from build123d import *

# Parameters (mm, degrees)
F1_DEPTH    = 10
F2_T1_DEPTH = 10
F2_T3_DEPTH = 20


# Not quite as in the source:
# - a fillet or chamfer that OpenCascade refuses, or shapes differently, is made with other operations: its cross-section is extruded or revolved along the edge and cut away or added
# - a feature names something its author has since deleted; it is built from what else it names


with BuildPart() as f1:
    # F0 (on Right) → F1 (new body)
    with BuildSketch(Plane.YZ):
        with BuildLine():
            Line((20, 0), (0, 0))
            Line((0, 0), (0, -3))
            Line((0, -3), (15, -3))
            ThreePointArc((15, -3), (36.9203102168, 6.0796897832), (46, 28))
            ThreePointArc((46, 28), (44.5, 29.5), (43, 28))
            ThreePointArc((43, 28), (37.1421356237, 13.8578643763), (23, 8))
            Line((23, 8), (23, 18))
            ThreePointArc((23, 18), (21.5, 19.5), (20, 18))
            Line((20, 18), (20, 8))
            Line((20, 8), (0, 8))
            Line((0, 8), (0, 5))
            Line((0, 5), (20, 5))
            Line((20, 5), (20, 0))
        make_face()
        with BuildLine():
            Line((23, 0.1252802705), (23, 6))
            ThreePointArc((23, 6), (30.9268806632, 7.4777057094), (37.7888888889, 11.712312459))
            ThreePointArc((37.7888888889, 11.712312459), (38.4580316617, 11.7150853421), (38.5307017544, 11.0498945447))
            ThreePointArc((38.5307017544, 11.0498945447), (31.6848160775, 4.2804529457), (23, 0.1252802705))
        make_face(mode=Mode.SUBTRACT)
    extrude(amount=F1_DEPTH)

    # F2: fillet of radius 2 on 8 edges, made by hand

    # F2_s2 → F2_t1 (join)
    with BuildSketch(Plane.YZ):
        with BuildLine():
            ThreePointArc((20, 10), (19.4142135624, 8.5857864376), (18, 8))
            Line((18, 8), (20, 8))
            Line((20, 8), (20, 10))
        make_face()
        with BuildLine():
            ThreePointArc((25.2222222222, 8.1238402), (23.6666666667, 8.620744195), (23, 10.11145618))
            Line((23, 10.11145618), (23, 8))
            ThreePointArc((23, 8), (24.1128351181, 8.0309840503), (25.2222222222, 8.1238402))
        make_face()
        with BuildLine():
            ThreePointArc((23, 4.0834785138), (23.5280398556, 5.4374849146), (24.8333333333, 6.076521971))
            ThreePointArc((24.8333333333, 6.076521971), (23.9174648117, 6.0191388176), (23, 6))
            Line((23, 6), (23, 4.0834785138))
        make_face()
        with BuildLine():
            ThreePointArc((25.7407407407, 1.0623592655), (23.8778327846, 1.2646093225), (23, 2.920127592))
            Line((23, 2.920127592), (23, 0.1252802705))
            ThreePointArc((23, 0.1252802705), (24.3820770695, 0.5595803629), (25.7407407407, 1.0623592655))
        make_face()
    extrude(amount=F2_T1_DEPTH)

    # F2_s4 → F2_t3 (cut)
    with BuildSketch(Plane.YZ.offset(-5)):
        with BuildLine():
            ThreePointArc((2, 8), (0.5857864376, 7.4142135624), (0, 6))
            Line((0, 6), (0, 8))
            Line((0, 8), (2, 8))
        make_face()
        with BuildLine():
            ThreePointArc((0, 7), (0.5857864376, 5.5857864376), (2, 5))
            Line((2, 5), (0, 5))
            Line((0, 5), (0, 7))
        make_face()
        with BuildLine():
            ThreePointArc((2, 0), (0.5857864376, -0.5857864376), (0, -2))
            Line((0, -2), (0, 0))
            Line((0, 0), (2, 0))
        make_face()
        with BuildLine():
            ThreePointArc((0, -1), (0.5857864376, -2.4142135624), (2, -3))
            Line((2, -3), (0, -3))
            Line((0, -3), (0, -1))
        make_face()
    extrude(amount=F2_T3_DEPTH, mode=Mode.SUBTRACT)


solid = f1.part
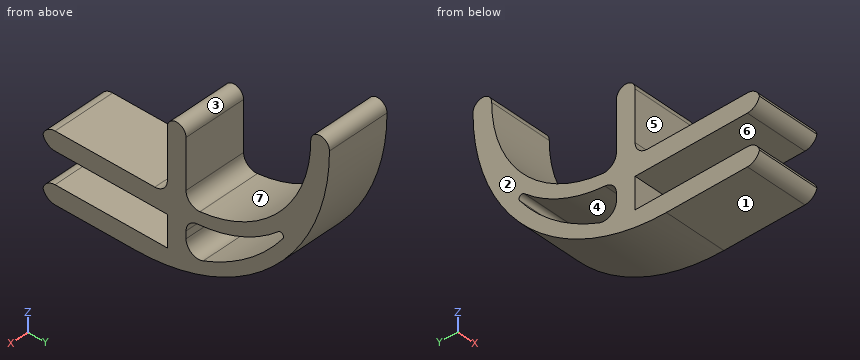
Part model, mm, in its own coordinate system. Face numbers are marked on the shaded views. A direction names the side the tool comes from. Give positions to 0.01 mm unless a question says otherwise; leave off trailing zeros. Order: outer loops, then holes, each group sorted by start corner. A loop starts at its lowest first (then second) coordinate and runs counter-clockwise, first axis right, second up. Notation, with made-up numbers: (36.5, 10.5) -> (75.5, 10.5) arc R21 ccw to (75.5, 21.5) -> close; hole circle Ø6 at (-4, -18). An arc over 180 degrees is marked (long way). Use one line per item in the form item = value.
(1) Saw through at C-C (z = 9.5). Write the cut outline in (x, y), then the cut area to 3 significant figures.
Solution:
outline = (0, 19.94) -> (10, 19.94) -> (10, 23.1) -> (0, 23.1) -> close; (0, 30.6) -> (10, 30.6) -> (10, 34.91) -> (0, 34.91) -> close; (0, 37.33) -> (10, 37.33) -> (10, 39.87) -> (0, 39.87) -> close
area = 100 mm²
(2) Saw through at B-B (x = 4.75). Write the cut outline in (y, z) (1 decimal), then the cut area to 3 significant figures.
Solution:
outline = (0.1, -1.5) arc R2 ccw to (2, -3) -> (15, -3) arc R31 ccw to (46, 28) arc R1.5 ccw to (43, 28) arc R20 cw to (25.2, 8.1) arc R2 cw to (23, 10.1) -> (23, 18) arc R1.5 ccw to (20, 18) -> (20, 10) arc R2 cw to (18, 8) -> (2, 8) arc R2 ccw to (0.1, 6.5) arc R2 ccw to (2, 5) -> (20, 5) -> (20, 0) -> (2, 0) arc R2 ccw to start; hole (23, 2.9) arc R2 ccw to (25.7, 1.1) arc R29 ccw to (38.5, 11) arc R0.5 ccw to (37.8, 11.7) arc R22 cw to (24.8, 6.1) arc R2 ccw to (23, 4.1) -> close
area = 326 mm²
(3) Flat gauge pins, fed straight in: P1, Ø5, axis at x = 4.5, z = 17, coming from the -Y side; P2, Ø0.9, axis at x = 3, z = 3.5, coming from the +Y side; P3, Ø3, axis at x = 7.5, y = 22, coming from the +Z side. Where does each tip first touch, or does it go through?
Solution:
P1 = 20
P2 = 34.56
P3 = 19.5
(4) Tool access for the marked faces 5, 6 and 7: list every direction of +Z, -Z, +X, -X, +Y, -Y with a clear straight run to the whole face (end or side of a thin tool).
Solution:
face_5 = +Z, +X, -X, -Y
face_6 = +X, -X, -Y
face_7 = +Z, +X, -X
(5) Saw through at A-A (y = 5). Write the cut outline in (x, z).
Solution:
outline = (0, -3) -> (10, -3) -> (10, 0) -> (0, 0) -> close; (0, 5) -> (10, 5) -> (10, 8) -> (0, 8) -> close
(6) Drill centre lines: line 1 (Z direction, x = 0.5, y = 15.5); line 2 (Z direction, x = 8.5, y = 26); line 3 (Y direction, x = 1.5, z = 12). Where is each one in solid material? Low to high. Write a range as from..to.
Solution:
line_1 = -3..0, 5..8
line_2 = -0.98..1.17, 6.21..8.23
line_3 = 20..23, 35..41.55
(7) Pull direction Z, two halves, no side cores. Call the marked faces 1, 2, 3 and 4: +Z half, -Z half, draft (parallel to the pull), parting line (faces both ways), or undercut.
Solution:
face_1 = -Z half
face_2 = draft
face_3 = +Z half
face_4 = undercut
(8) Saw through at D-D (y = 29.5). Write the cut outline in (x, z), then the cut area to 3 significant figures.
Solution:
outline = (0, 0.6) -> (10, 0.6) -> (10, 2.89) -> (0, 2.89) -> close; (0, 6.98) -> (10, 6.98) -> (10, 9.09) -> (0, 9.09) -> close
area = 43.9 mm²
